Could you check a few things on this model? Use its own coordinates, in mm. Face numbers are marked on the shaded views. A direction names the side the tool comes from. Coordinates: 2 decimals unless noted, no trailing zeros. Write each loop counter-clockwise with the first axis right and the second up, starting at its lowest first coordinate (ties: lowest second). Pieces come first, ordered by that corner, then holes.
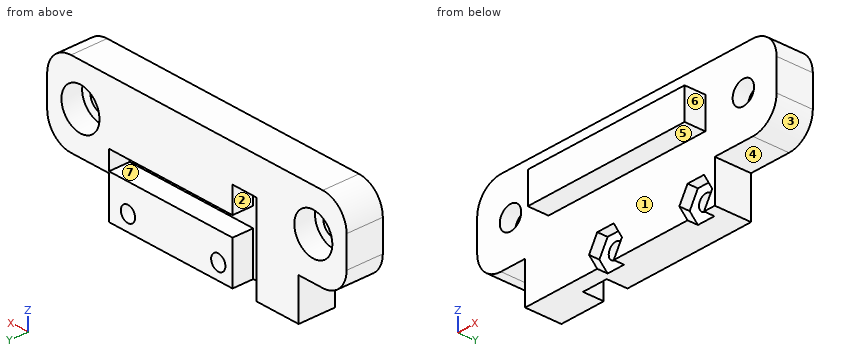
```python
from build123d import *

# Parameters (mm, degrees)
SKETCH_1_W          = 63
SKETCH_1_H          = 16
SKETCH_1_W_2        = 39.904611507
SKETCH_1_H_2        = 8
EXTRUDE_1_DEPTH     = 7
SKETCH_2_R          = 2.25
CUT_EXTRUDE_1_DEPTH = 47
SKETCH_3_W          = 33
SKETCH_3_H          = 6
EXTRUDE_2_DEPTH     = 4
SKETCH_5_W          = 26
SKETCH_5_H          = 3.69
CUT_EXTRUDE_2_DEPTH = 4
SKETCH_5_3_R        = 1.5
CUT_EXTRUDE_3_DEPTH = 20
CUT_EXTRUDE_4_DEPTH = 2
FILLET_1_R          = 5
SKETCH_7_R          = 4
CUT_EXTRUDE_5_DEPTH = 4


with BuildPart() as part:
    # Sketch 1 → Extrude 1 (new body)
    with BuildSketch(Plane(origin=(0, 0, 0), x_dir=(1, 0, 0), z_dir=(0, 1, 0))):
        with Locations((31.5, 8)):
            Rectangle(SKETCH_1_W, SKETCH_1_H)
        with Locations((30.047694247, 20)):
            Rectangle(SKETCH_1_W_2, SKETCH_1_H_2)
    extrude(amount=EXTRUDE_1_DEPTH)

    # Sketch 2 → Cut-Extrude 1 (cut)
    with BuildSketch(Plane(origin=(0, 0, 0), x_dir=(1, 0, 0), z_dir=(0, 1, 0))):
        with Locations(Location((7, 8, 0), (0, 0, 90))):
            Circle(SKETCH_2_R)
        with Locations(Location((56, 8, 0), (0, 0, 90))):
            Circle(SKETCH_2_R)
    extrude(amount=CUT_EXTRUDE_1_DEPTH, mode=Mode.SUBTRACT)

    # Sketch 3 → Extrude 2 (add)
    with BuildSketch(Plane.XZ):
        with Locations((31.5, -8)):
            Rectangle(SKETCH_3_W, SKETCH_3_H)
    extrude(amount=EXTRUDE_2_DEPTH)

    # Sketch 5 → Cut-Extrude 2 (cut)
    with BuildSketch(Plane(origin=(0, 7, 0), x_dir=(1, 0, 0), z_dir=(0, 1, 0))):
        with Locations((37, 13.845)):
            Rectangle(SKETCH_5_W, SKETCH_5_H)
        Polygon((24, 12), (24, 15.69), (24, 24), (19, 24), (19, 7), (24, 7), align=None)
    extrude(amount=-CUT_EXTRUDE_2_DEPTH, mode=Mode.SUBTRACT)

    # Sketch 5_3 → Cut-Extrude 3 (cut)
    with BuildSketch(Plane(origin=(0, 7, 0), x_dir=(1, 0, 0), z_dir=(0, 1, 0))):
        with Locations(Location((27, 21, 0), (0, 0, 270))):
            Circle(SKETCH_5_3_R)
        with Locations(Location((46, 21, 0), (0, 0, 270))):
            Circle(SKETCH_5_3_R)
    extrude(amount=-CUT_EXTRUDE_3_DEPTH, mode=Mode.SUBTRACT)

    # Sketch 6 → Cut-Extrude 4 (cut)
    with BuildSketch(Plane.XZ):
        Polygon((47.732050808, -18), (44.267949192, -18), (42.535898385, -21), (44.267949192, -24), (47.732050808, -24), (49.464101615, -21), align=None)
        Polygon((30.464101615, -21), (28.732050808, -18), (25.267949192, -18), (23.535898385, -21), (25.267949192, -24), (28.732050808, -24), align=None)
    extrude(amount=-CUT_EXTRUDE_4_DEPTH, mode=Mode.SUBTRACT)

    # Fillet 1
    fillet_1_edges = [part.edges().sort_by_distance(p)[0] for p in [
        (0, 3.5, 0),
        (0, 3.5, -16),
        (63, 3.5, -16),
        (63, 3.5, 0),
    ]]
    fillet(fillet_1_edges, radius=FILLET_1_R)

    # Sketch 7 → Cut-Extrude 5 (cut)
    with BuildSketch(Plane(origin=(0, 7, 0), x_dir=(1, 0, 0), z_dir=(0, 1, 0))):
        with Locations(Location((7, 8, 0), (0, 0, 270))):
            Circle(SKETCH_7_R)
        with Locations(Location((56, 8, 0), (0, 0, 270))):
            Circle(SKETCH_7_R)
    extrude(amount=-CUT_EXTRUDE_5_DEPTH, mode=Mode.SUBTRACT)


solid = part.part
```
1. I want a section at B-B on y = 5. Please give me the cut outline in (x, z).
Verdict:
outline: (0, -11) arc R5 ccw to (5, -16) - (10.1, -16) - (10.1, -24) - (19, -24) - (19, -7) - (24, -7) - (24, -12) - (50, -12) - (50, -15.69) - (24, -15.69) - (24, -24) - (50, -24) - (50, -16) - (58, -16) arc R5 ccw to (63, -11) - (63, -5) arc R5 ccw to (58, 0) - (5, 0) arc R5 ccw to (0, -5) - close; hole circle Ø8 at (7, -8); hole circle Ø3 at (27, -21); hole circle Ø3 at (46, -21); hole circle Ø8 at (56, -8)
2. I want a section at C-C on x = 41.5. Please give me the cut outline in (y, z), plus the area to 3 significant figures.
Verdict:
outline: (-4, -11) - (0, -11) - (0, -24) - (7, -24) - (7, -15.69) - (3, -15.69) - (3, -12) - (7, -12) - (7, 0) - (0, 0) - (0, -5) - (-4, -5) - close
area: 177 mm2
3. I want a section at D-D on x = 27. Please give me the cut outline in (y, z).
Verdict:
outline: (-4, -11) - (0, -11) - (0, -18) - (2, -18) - (2, -19.5) - (7, -19.5) - (7, -15.69) - (3, -15.69) - (3, -12) - (7, -12) - (7, 0) - (0, 0) - (0, -5) - (-4, -5) - close; (2, -24) - (7, -24) - (7, -22.5) - (2, -22.5) - close
4. Please list where these lines run through material, in increasing order: line 1 along X through (y, z) = (0.8, -8); line 2 along X through (y, z) = (6.25, -8.25); line 3 along X through (y, z) = (6.25, -22.75).
Verdict:
line 1: x = 0 to 4.75, 9.25 to 53.75, 58.25 to 63
line 2: x = 0 to 3.01, 10.99 to 19, 24 to 52.01, 59.99 to 63
line 3: x = 10.1 to 19, 24 to 50
5. If we mould it in two halves opening along X, with no side actions, what happens to the marked faces 1, 2 and 3? For each: pulls with the +X half, pulls with the -X half, needs draft (parallel to the pull), parting line crosses it, or undercut.
Verdict:
face 1: needs draft
face 2: undercut
face 3: pulls with the +X half
6. I want a section at A-A on x = 7. Please give me the cut outline in (y, z), plus the area to 3 significant figures.
Verdict:
outline: (0, -16) - (7, -16) - (7, -12) - (3, -12) - (3, -10.25) - (0, -10.25) - close; (0, -5.75) - (3, -5.75) - (3, -4) - (7, -4) - (7, 0) - (0, 0) - close
area: 66.5 mm2
7. On a 3-axis mill with a long thin cutter (end or side, diameter ignored), from which of +Z, -Z, +X, -X, +Y, -Y can I reach the whole of each face in a straight line? I mean the marked faces 4, 5, 6 and 7. Say none if no direction works.
Verdict:
face 4: -Z, +X, +Y, -Y
face 5: -Z, +X, -X, -Y
face 6: +Z, -Z, +X, -Y
face 7: +Y
8. For pin 1 (4 mm diameter, centred on y = 4.5, z = -14, fed in from -X); pin 2 (3.5 mm diameter, centred on x = 46, z = -21, fed in from -Y); pin 3 (1.5 mm diameter, centred on y = 4.5, z = -19, fed in from -X), each with a flat end and sliding along its axis, tell me the tip position at first contact or that it passes through.
Verdict:
pin 1: stops at x = 0.1
pin 2: stops at y = 2
pin 3: stops at x = 10.1
